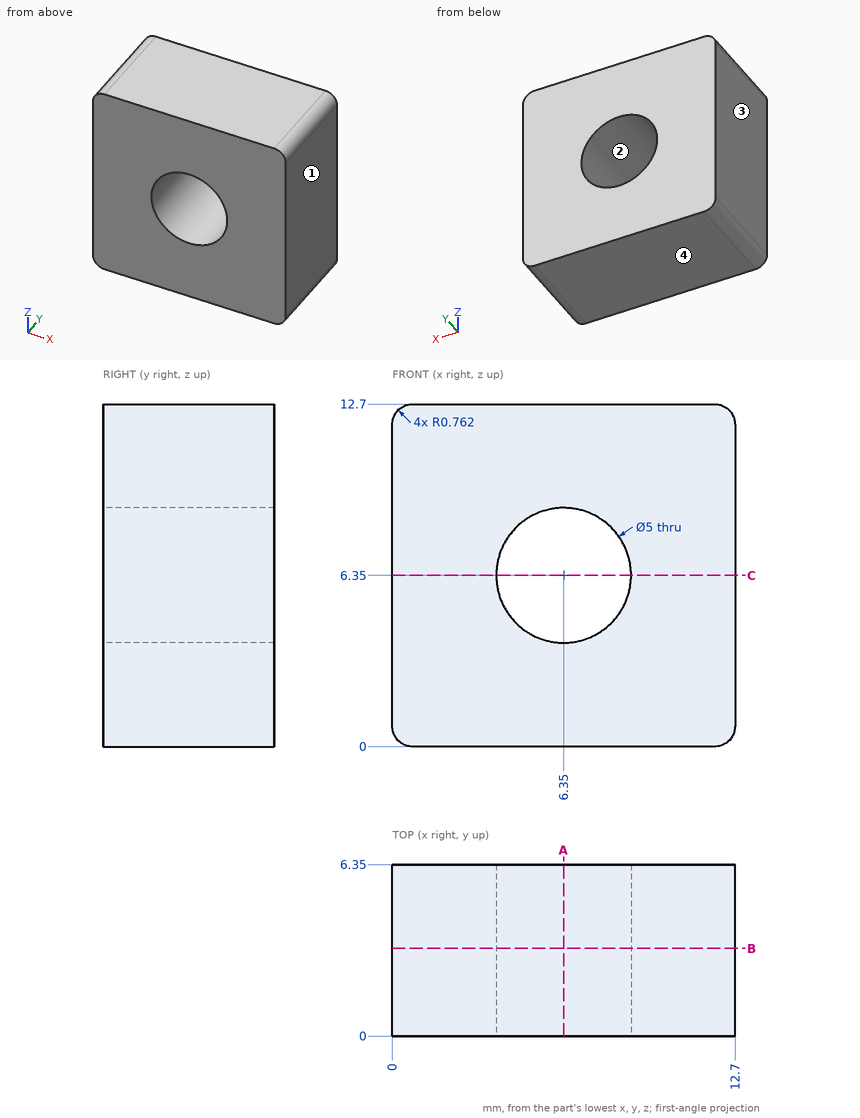
Source: three-view drawing plus pictorial views. Frame: mm from the lowest corner of the part. Give positions to 0.01 mm unless a question says otherwise; leave off trailing zeros. Order: outer loops, then holes, each group sorted by start corner. A loop starts at its lowest first (then second) coordinate and runs counter-clockwise, first axis right, second up. Notation, with made-up numbers: (4, -30.5) -> (28, -30.5) arc R6 ccw to (28, -19.5) -> close; hole circle Ø2 at (81.25, 76). An arc over 180 degrees is marked (long way). Write each question's results on one line, items separated by ' | '. Start each with the question number.
Item 1: Cut plane A-A on x = 6.35. Return the cut outline in (y, z).
Item 2: Cut plane C-C on z = 6.35. Return the cut outline in (x, y).
Item 3: Mould query, pull axis X, two halves, no side actions, for the marked faces 1, 2, 3 and 4. Classes: pulls with the +X half, pulls with the -X half, needs draft (parallel to the pull), parting line crosses it, or undercut.
Item 4: Cut plane B-B on y = 3.25. Return the cut outline in (x, z).
Item 5: Contact query for flat-ended pins moving along their axis: P1, Ø4, axis at x = 6.35, z = 6.35, coming from the -Y side; P2, Ø4, axis at x = 6.5, z = 8.5, coming from the +Y side. Output: stop coordinate, or through.
Item 6: Line query: line 1 (Z direction, x = 6.35, y = 3.25); line 2 (X direction, y = 4.75, z = 4.75); line 3 (Z direction, x = 5, y = 1). Output: solid intervals per line, ascending.
Established:
1) outline: (0, 0) -> (6.35, 0) -> (6.35, 3.85) -> (0, 3.85) -> close; (0, 8.85) -> (6.35, 8.85) -> (6.35, 12.7) -> (0, 12.7) -> close
2) outline: (0, 0) -> (3.85, 0) -> (3.85, 6.35) -> (0, 6.35) -> close; (8.85, 0) -> (12.7, 0) -> (12.7, 6.35) -> (8.85, 6.35) -> close
3) face 1: pulls with the +X half | face 2: undercut | face 3: pulls with the -X half | face 4: needs draft
4) outline: (0, 0.76) arc R0.76 ccw to (0.76, 0) -> (11.94, 0) arc R0.76 ccw to (12.7, 0.76) -> (12.7, 11.94) arc R0.76 ccw to (11.94, 12.7) -> (0.76, 12.7) arc R0.76 ccw to (0, 11.94) -> close; hole circle Ø5 at (6.35, 6.35)
5) P1: through | P2: y = 6.35
6) line 1: 0 to 3.85, 8.85 to 12.7 | line 2: 0 to 4.43, 8.27 to 12.7 | line 3: 0 to 4.25, 8.45 to 12.7
